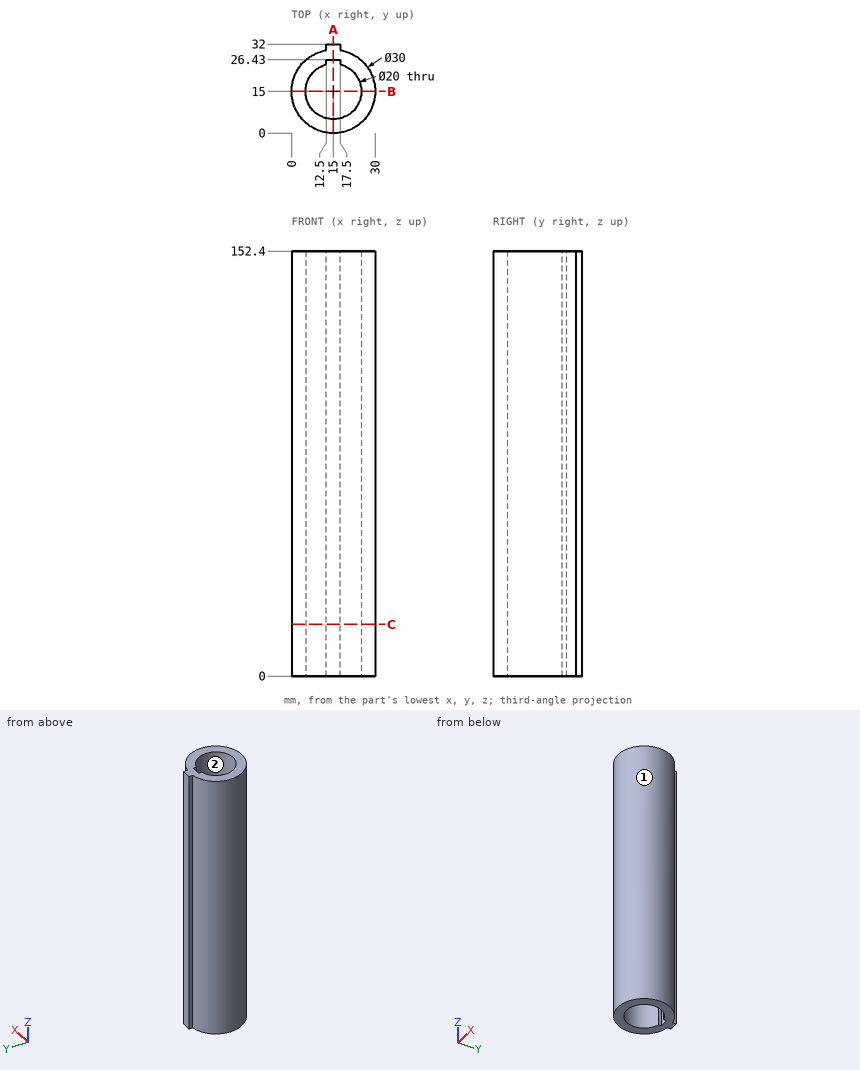
Could you check a few things on this drawing? It's one solid part, dimensions in mm from its lowest x, y, z. Give positions to 0.01 mm unless a question says otherwise; leave off trailing zeros. Order: outer loops, then holes, each group sorted by start corner. A loop starts at its lowest first (then second) coordinate and runs counter-clockwise, first axis right, second up. Notation, with made-up numbers: (23, 35) - (45, 35) arc R14 ccw to (45, 43) - close; hole circle Ø6 at (51, 66). An arc over 180 degrees is marked (long way). Return JSON: item names as keys, results as strings. Group by question number.
Q1. Thinking about a two-plate mould opening in X: for the marked faces 1 and 2, which applies, pulls with the +X half, pulls with the -X half, needs draft (parallel to the pull), parting line crosses it, or undercut?
Q2. Suppose I cut it at A-A, the plane x = 15. Please give me the cut outline in (y, z), and give its area (3 significant figures).
Q3. Suppose I cut it at B-B, the plane y = 15. Please give me the cut outline in (x, z).
Q4. Please list where these lines run through material, in increasing order: line 1 along X through (y, z) = (15, 71); line 2 along Y through (x, z) = (15, 53.5); line 3 along X through (y, z) = (31.5, 98). Write a range as [from, to].
Q5. Suppose I cut it at C-C, the plane z = 18.5. Please give me the cut outline in (x, y), and give its area (3 significant figures).
Q6. Will these pins go through, and if not, where does the flat tip stop? pin 1 Ø1.5 at (x, y) = (27, 4.5) entering from +Z; pin 2 Ø4 at (x, z) = (25, 85.5) entering from -Y; pin 3 Ø2.5 at (y, z) = (31.5, 90) entering from +X; pin 4 Ø0.5 at (y, z) = (25, 66) entering from +X.
Resolved:
{
 "1": {"face 1": "parting line crosses it", "face 2": "undercut"},
 "2": {"outline": "(0, 0) - (5, 0) - (5, 152.4) - (0, 152.4) - close; (26.43, 0) - (32, 0) - (32, 152.4) - (26.43, 152.4) - close", "area": "1,610 mm2"},
 "3": {"outline": "(0, 0) - (5, 0) - (5, 152.4) - (0, 152.4) - close; (25, 0) - (30, 0) - (30, 152.4) - (25, 152.4) - close"},
 "4": {"line 1": "x = [0, 5], [25, 30]", "line 2": "y = [0, 5], [26.43, 32]", "line 3": "x = [12.5, 17.5]"},
 "5": {"outline": "(12.5, 29.79) arc R15 ccw (long way) to (17.5, 29.79) - (17.5, 32) - (12.5, 32) - close; hole (12.5, 24.68) arc R10 ccw (long way) to (17.5, 24.68) - (17.5, 26.43) - (12.5, 26.43) - close", "area": "395 mm2"},
 "6": {"pin 1": "passes through", "pin 2": "stops at y = 2.31", "pin 3": "stops at x = 17.5", "pin 4": "stops at x = 26.4"}
}
